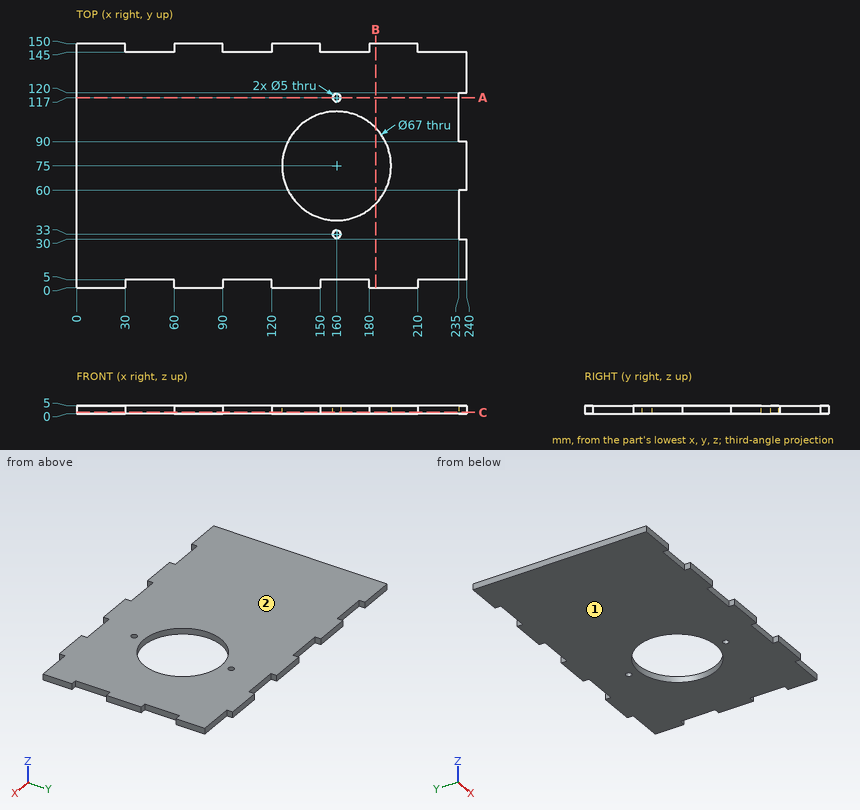
Here's the drawing with two shaded views (mm, measured from the low corner). I have some questions. Give positions to 0.01 mm unless a question says otherwise; leave off trailing zeros. Loops run counter-clockwise (first coordinate to the right, second up) from the corner with the lowest first, then second, coordinate; pieces in that order, holes last. Notation, with made-up numbers: (61.25, 40.25) -> (111.25, 40.25) arc R19 cw to (111.25, 49.25) -> close; hole circle Ø8 at (6, 21.5). An arc over 180 degrees is marked (long way). Use one line per item in the form item = value.
1) I need wall thicknesses on line 1 along Y through (x, z) = (160, 1.9); line 2 along X through (y, z) = (33, 1.6); line 3 along X through (y, z) = (80, 4.55). Which ranges of each line are inside material? Lowest first, please.
Answers:
line_1 = 5 to 30.5, 35.5 to 41.5, 108.5 to 114.5, 119.5 to 145
line_2 = 0 to 157.5, 162.5 to 235
line_3 = 0 to 126.88, 193.12 to 240
2) Will these pins go through, and if not, where does the flat tip stop? pin 1 (2.5 mm diameter, centred on x = 162, z = 1.5, fed in from -Y); pin 2 (2.5 mm diameter, centred on x = 48.5, z = 2, fed in from +Y); pin 3 (3 mm diameter, centred on y = 49.5, z = 4.5, fed in from +X); pin 4 (4 mm diameter, centred on x = 160, y = 33, fed in from +Z).
Answers:
pin_1 = 5
pin_2 = 145
pin_3 = 235
pin_4 = through
3) If we section it at B-B (x = 184): Please give me the cut outline in (y, z).
Answers:
outline = (0, 0) -> (51.63, 0) -> (51.63, 5) -> (0, 5) -> close; (98.37, 0) -> (150, 0) -> (150, 5) -> (98.37, 5) -> close
4) If we section it at A-A (y = 117): Please give me the cut outline in (x, z), plus the area to 3 significant figures.
Answers:
outline = (0, 0) -> (157.5, 0) -> (157.5, 5) -> (0, 5) -> close; (162.5, 0) -> (235, 0) -> (235, 5) -> (162.5, 5) -> close
area = 1,150 mm²
5) If we section it at C-C (z = 0.95): Count the separate pieces of the cut face and the enclosed holes in it, plus the area to 3 significant figures.
Answers:
separate_pieces = 1
enclosed_holes = 3
area = 30,900 mm²
6) We'd pull the mould along Z, two halves only. Please class the marked faces 1 and 2: released by +Z, released by -Z, zero draft, split by the parting line, or undercut.
Answers:
face_1 = released by -Z
face_2 = released by +Z
